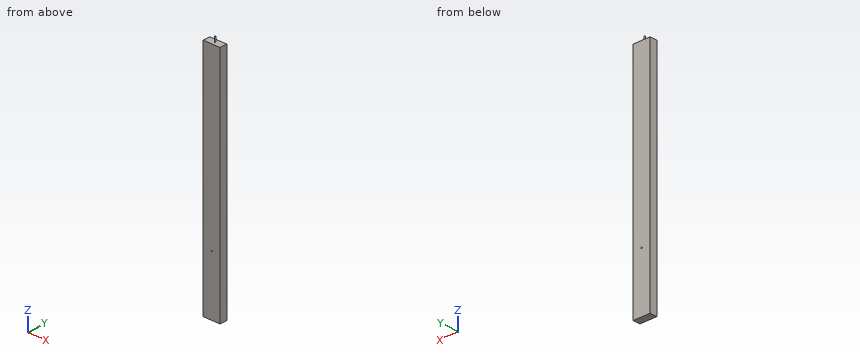
from build123d import *

# Parameters (mm, degrees)
F0_W     = 88.9
F0_H     = 1219.2
F1_DEPTH = 38.1
F3_D     = 6.35
F4_R     = 2.54
F5_DEPTH = 25.4


with BuildPart() as f1:
    # F0 (on Front) → F1 (new body)
    with BuildSketch(Plane.XZ):
        with Locations((-44.45, 609.6)):
            Rectangle(F0_W, F0_H)
    extrude(amount=F1_DEPTH)

    # F3 (through all)
    with Locations(Plane.XZ.offset(38.1)):
        with Locations((-44.45, 304.8)):
            Hole(F3_D / 2)

    # F4 (on face) → F5 (join)
    with BuildSketch(Plane.XY.offset(1219.2)):
        with Locations((-44.45, -18.403284)):
            Circle(F4_R)
    extrude(amount=F5_DEPTH)


solid = f1.part
Part model, mm, in its own coordinate system. Coordinates: 2 decimals unless noted, no trailing zeros. Order: outer loops, then holes, each group sorted by start corner. A loop starts at its lowest first (then second) coordinate and runs counter-clockwise, first axis right, second up. Notation, with made-up numbers: M 70.25,12 L 123.25,12 A15 ccw 123.25,20 Z; hole C 53.25,20.5 d10. An arc over 180 degrees is marked long. Use a Markdown table: item, result.
(1) Probe L1, parallel to X at y = -27, z = 304; L2, parallel to X at y = -13, z = 304.8 (3 decimals); L3, parallel to Z at x = -44, y = -13. List the from-to ranges inside material, lowest first.
A:
| item | result |
|---|---|
| L1 | x = -88.9 to -47.52, -41.38 to 0 |
| L2 | x = -88.9 to -47.625, -41.275 to 0 |
| L3 | z = 0 to 301.66, 307.94 to 1219.2 |
(2) Flat gauge pin, fed straight in: pin 1 (1 mm diameter, centred on x = -35, y = -24.5, fed in from +Z). Where does the tip first touch, or does it go through?
A:
| item | result |
|---|---|
| pin 1 | stops at z = 1219.2 |
(3) Cut at A-A on x = -28. Write the cut outline in (y, z), then the cut area to 3 significant figures.
A:
| item | result |
|---|---|
| outline | M -38.1,0 L 0,0 L 0,1219.2 L -38.1,1219.2 Z |
| area | 46,500 mm^2 |
